Check sheet for the modelled part. Datum: model origin and axes. Units: mm. Face numbers are marked on the shaded views. A direction names the side the tool comes from. Coordinates: 2 decimals unless noted, no trailing zeros. Loops run counter-clockwise (first coordinate to the right, second up) from the corner with the lowest first, then second, coordinate; pieces in that order, holes last. Notation, with made-up numbers: (35.25, 43.5) - (63.25, 43.5) arc R18 cw to (63.25, 55.5) - close; hole circle Ø8 at (75.5, -4). An arc over 180 degrees is marked (long way). Answer as a JSON object with one key per item and string values. Group by question number.
from build123d import *

# Parameters (mm, degrees)
SKETCH1_R           = 2.5
BOSS_EXTRUDE1_DEPTH = 13
BOSS_EXTRUDE2_DEPTH = 4


with BuildPart() as part:
    # Sketch1 → Boss-Extrude1 (new body)
    with BuildSketch(Plane(origin=(0, 0, 0), x_dir=(1, 0, 0), z_dir=(0, 1, 0))):
        with Locations(Location((0, 0, 0), (0, 0, 90))):
            Circle(SKETCH1_R)
    extrude(amount=BOSS_EXTRUDE1_DEPTH)

    # Sketch2 → Boss-Extrude2 (add)
    with BuildSketch(Plane(origin=(0, 13, 0), x_dir=(1, 0, 0), z_dir=(0, 1, 0))):
        Polygon((5, 0), (2.5, 4.330127019), (-2.5, 4.330127019), (-5, 0), (-2.5, -4.330127019), (2.5, -4.330127019), align=None)
    extrude(amount=-BOSS_EXTRUDE2_DEPTH)

    # Sketch3 → Cut-Revolve1 (revolve, cut)
    with BuildSketch(Plane.XY, mode=Mode.PRIVATE) as cut_revolve1_sk:
        Polygon((4, 13), (5, 12), (5, 13), align=None)
    revolve(cut_revolve1_sk.sketch.rotate(Axis((0, 0, 0), (0, 1, 0)), 90), axis=Axis((0, 0, 0), (0, 1, 0)), mode=Mode.SUBTRACT)


solid = part.part
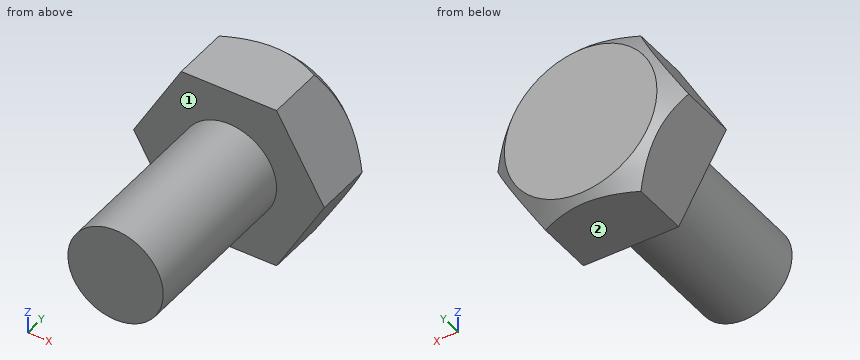
1. Gauge pin test, flat ends, axial feed: pin 1 (1 mm diameter, centred on x = -2.5, y = 5.5, fed in from -Z); pin 2 (2.5 mm diameter, centred on x = 2.5, z = -1, fed in from -Y); pin 3 (6 mm diameter, centred on x = 2, y = 5, fed in from -Z); pin 4 (4 mm diameter, centred on x = -3, y = 3.5, fed in from -Z). Record the tip position at first contact, or that the pin passes through.
2. Material ranges on line 1 (Y direction, x = -3, z = 0.25); line 2 (Z direction, x = 1, y = 7), recorded low to high.
3. Sectioned sample at B-B on y = 1. Record the cut outline in (x, z).
4. Sectioned sample at A-A on x = 0. Record the cut outline in (y, z).
5. Access from +Z, -Z, +X, -X, +Y, -Y to the whole of each face (thin tool, end or side, straight path). Record for the marked faces 1 and 2.
Answers follow:
{
 "1": {"pin 1": "stops at z = -1.5", "pin 2": "stops at y = 0", "pin 3": "stops at z = -2.5", "pin 4": "stops at z = -2.29"},
 "2": {"line 1": "y = 9 to 13", "line 2": "z = -2.29 to 2.29"},
 "3": {"outline": "circle Ø5 at (0, 0)"},
 "4": {"outline": "(0, -2.5) - (9, -2.5) - (9, -4.33) - (12.67, -4.33) - (13, -4) - (13, 4) - (12.67, 4.33) - (9, 4.33) - (9, 2.5) - (0, 2.5) - close"},
 "5": {"face 1": "-Y", "face 2": "-Z, +X, -X, +Y, -Y"}
}
